Geometry check sheet. Reference: the model listing, model coordinates, mm. Coordinates: 2 decimals unless noted, no trailing zeros. Order: outer loops, then holes, each group sorted by start corner. A loop starts at its lowest first (then second) coordinate and runs counter-clockwise, first axis right, second up. Notation, with made-up numbers: (39.25, 27.5) - (93.25, 27.5) arc R26 cw to (93.25, 52.5) - close; hole circle Ø2 at (44, 88). An arc over 180 degrees is marked (long way). Use CSV: the item, a comma, the result in double quotes. Start each with the question number.
1) Depth check by flat-ended pin: P1, Ø4.5, axis at x = -12.7, y = 482.6, coming from the -Z side. Enter the tip coordinate at first touch or a pass-through.
2) Sectioned sample at B-B, the plane y = 325. Record the cut outline in (x, z) (3 decimals), and give its area (3 significant figures).
3) Sectioned sample at C-C, the plane z = 0.9. Count the separate pieces of the cut face and the enclosed holes in it, and give its area (3 significant figures).
4) Thickness scan on probe 1 along X at (y, z) = (419, 2.15); probe 2 along Y at (x, z) = (-72.5, 2.3); probe 3 along X at (y, z) = (336, 1.85). Record the ranges inside material, lowest first. Write a range as [from, to].
5) Sectioned sample at A-A, the plane x = -205. Record the cut outline in (y, z) (3 decimals), and give its area (3 significant figures).
from build123d import *

# Parameters (mm, degrees)
SKETCH1_W              = 254
SKETCH1_H              = 711.2
BOSS_EXTRUDE1_DEPTH    = 3.175
F_10_CLEARANCE_HOLE1_D = 5.1054
LPATTERN1_COUNT        = 11
LPATTERN1_PITCH        = 63.5
SKETCH7_W              = 203.2
SKETCH7_H              = 50.8
CUT_EXTRUDE1_DEPTH     = 756.20296651


with BuildPart() as part:
    # Sketch1 → Boss-Extrude1 (new body)
    with BuildSketch(Plane.XY):
        with Locations((-127, 355.6)):
            Rectangle(SKETCH1_W, SKETCH1_H)
    extrude(amount=BOSS_EXTRUDE1_DEPTH)

    # #10 Clearance Hole1 (through all)
    with Locations(Plane.XY.offset(3.175)):
        with Locations((-241.3, 673.1), (-12.7, 673.1)):
            f_10_clearance_hole1 = Hole(F_10_CLEARANCE_HOLE1_D / 2)

    # LPattern1: #10 Clearance Hole1 ×11
    with Locations(*[(0, -i * LPATTERN1_PITCH, 0) for i in range(1, LPATTERN1_COUNT)]):
        add(f_10_clearance_hole1, mode=Mode.SUBTRACT)

    # Sketch7 → Cut-Extrude1 (cut, through all)
    with BuildSketch(Plane(origin=(0, 0, 0), x_dir=(-1, 0, 0), z_dir=(0, 0, -1))):
        with Locations((127, 330.2)):
            Rectangle(SKETCH7_W, SKETCH7_H)
    extrude(amount=-CUT_EXTRUDE1_DEPTH, mode=Mode.SUBTRACT)


solid = part.part
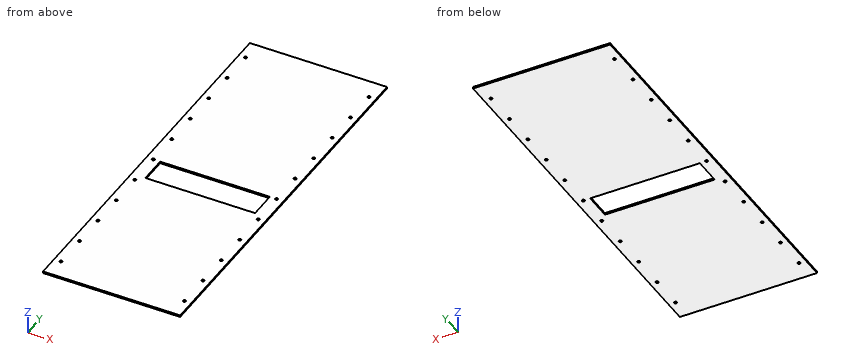
Evaluation:
1,P1,"through"
2,outline,"(-254, 0) - (-228.6, 0) - (-228.6, 3.175) - (-254, 3.175) - close; (-25.4, 0) - (0, 0) - (0, 3.175) - (-25.4, 3.175) - close"
2,area,"161 mm²"
3,separate pieces,"1"
3,enclosed holes,"23"
3,area,"170,000 mm²"
4,probe 1,"[-254, -243.85], [-238.75, -15.25], [-10.15, 0]"
4,probe 2,"[0, 304.8], [355.6, 711.2]"
4,probe 3,"[-254, -228.6], [-25.4, 0]"
5,outline,"(0, 0) - (304.8, 0) - (304.8, 3.175) - (0, 3.175) - close; (355.6, 0) - (711.2, 0) - (711.2, 3.175) - (355.6, 3.175) - close"
5,area,"2,100 mm²"
